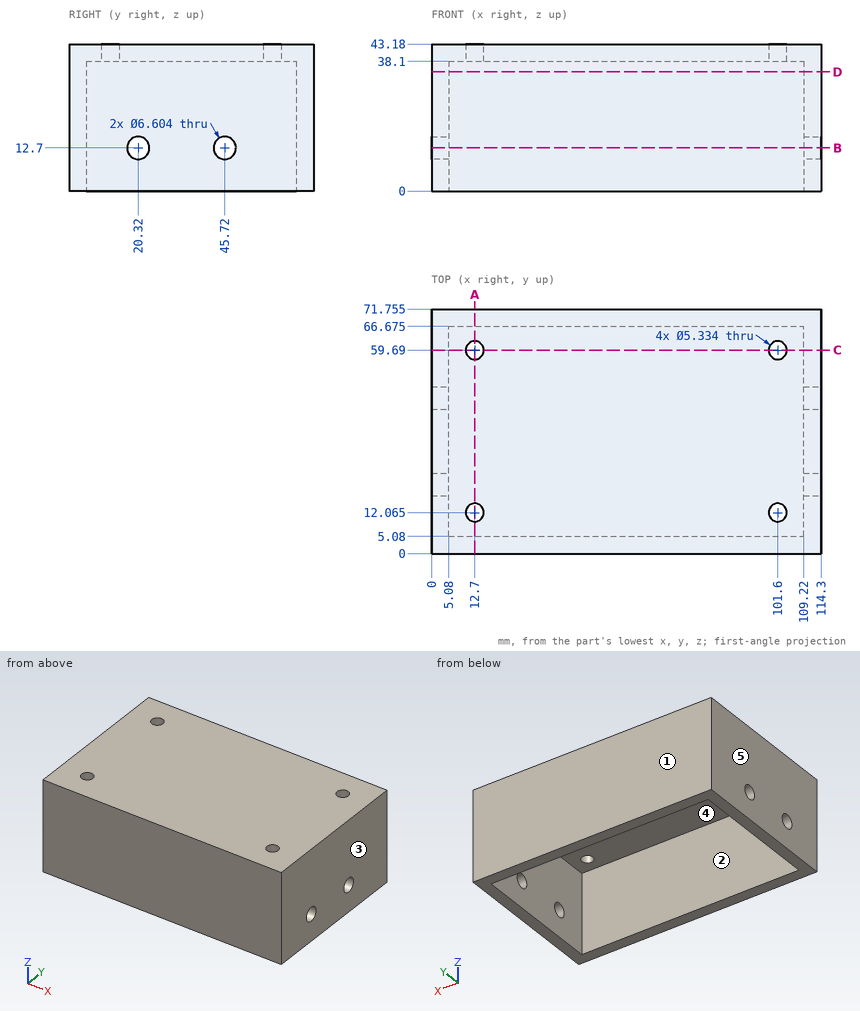
Verification items for this drawing (mm, ordinates from the low corner). A direction names the side the tool comes from. Give positions to 0.01 mm unless a question says otherwise; leave off trailing zeros. Loops run counter-clockwise (first coordinate to the right, second up) from the corner with the lowest first, then second, coordinate; pieces in that order, holes last. Notation, with made-up numbers: M 29.25,63 L 60.25,63 A23 cw 60.25,88 Z; hole C 81,7.25 d10. An arc over 180 degrees is marked long. Return JSON: item names as keys, results as strings. Group by question number.
1. Thickness scan on L1, parallel to Y at x = 1.2, z = 12.7 (3 decimals); L2, parallel to Y at x = 7, z = 19.5 (3 decimals); L3, parallel to X at y = 14.5, z = 23. Record the ranges inside material, lowest first.
2. Cross-section at A-A on x = 12.7. Record the boundary of the cut face in (y, z) (3 decimals).
3. Mould release check, pull along Y, two halves, no side actions. Record for the marked faces 1, 2 and 3: released by +Y, released by -Y, zero draft, split by the parting line, or undercut.
4. Cross-section at B-B on z = 12.7. Record the boundary of the cut face in (x, y) (3 decimals), plus the area to 3 significant figures.
5. Cross-section at C-C on y = 59.69. Record the boundary of the cut face in (x, z), plus the area to 3 significant figures.
6. Go/stop test with a flat-tipped pin: pin 1 (1 mm diameter, centred on x = 39.5, y = 15.5, fed in from -Z). Record where the tip stops, or that it passes through.
7. Tool access check on the marked faces 4 and 5. Record the directions out of +Z, -Z, +X, -X, +Y, -Y that give a thin tool (end or side, any length) a straight path to the whole face; none if there is none.
8. Cross-section at D-D on z = 35. Record the boundary of the cut face in (x, y) (3 decimals).
Return value:
{
 "1": {"L1": "0 to 17.018, 23.622 to 42.418, 49.022 to 71.755", "L2": "0 to 5.08, 66.675 to 71.755", "L3": "0 to 5.08, 109.22 to 114.3"},
 "2": {"outline": "M 0,0 L 5.08,0 L 5.08,38.1 L 9.398,38.1 L 9.398,43.18 L 0,43.18 Z; M 14.732,38.1 L 57.023,38.1 L 57.023,43.18 L 14.732,43.18 Z; M 62.357,38.1 L 66.675,38.1 L 66.675,0 L 71.755,0 L 71.755,43.18 L 62.357,43.18 Z"},
 "3": {"face 1": "released by +Y", "face 2": "undercut", "face 3": "zero draft"},
 "4": {"outline": "M 0,0 L 114.3,0 L 114.3,17.018 L 109.22,17.018 L 109.22,5.08 L 5.08,5.08 L 5.08,17.018 L 0,17.018 Z; M 0,23.622 L 5.08,23.622 L 5.08,42.418 L 0,42.418 Z; M 0,49.022 L 5.08,49.022 L 5.08,66.675 L 109.22,66.675 L 109.22,49.022 L 114.3,49.022 L 114.3,71.755 L 0,71.755 Z; M 109.22,23.622 L 114.3,23.622 L 114.3,42.418 L 109.22,42.418 Z", "area": "1,650 mm^2"},
 "5": {"outline": "M 0,0 L 5.08,0 L 5.08,38.1 L 10.03,38.1 L 10.03,43.18 L 0,43.18 Z; M 15.37,38.1 L 98.93,38.1 L 98.93,43.18 L 15.37,43.18 Z; M 104.27,38.1 L 109.22,38.1 L 109.22,0 L 114.3,0 L 114.3,43.18 L 104.27,43.18 Z", "area": "914 mm^2"},
 "6": {"pin 1": "z = 38.1"},
 "7": {"face 4": "-Z", "face 5": "+Z, -Z, -X, +Y, -Y"},
 "8": {"outline": "M 0,0 L 114.3,0 L 114.3,71.755 L 0,71.755 Z; hole M 5.08,5.08 L 109.22,5.08 L 109.22,66.675 L 5.08,66.675 Z"}
}
